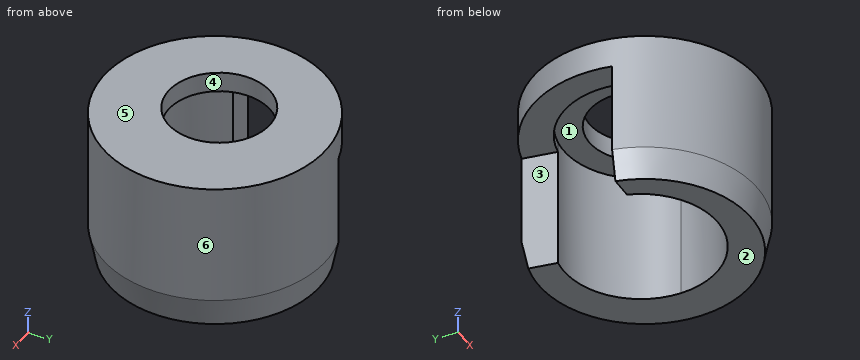
from build123d import *

# Parameters (mm, degrees)
F0_R     = 10.95
F1_DEPTH = 15
F3_DEPTH = 12
F4_DEPTH = 13
F6_D     = 10
F6_DEPTH = 10
F7_SIZE2 = 0.6
F7_SIZE  = 3


with BuildPart() as f1:
    # F0 (on Top) → F1 (new body)
    with BuildSketch(Plane.XY):
        Circle(F0_R)
    extrude(amount=F1_DEPTH)

    # F2 (on face) → F3 (cut)
    with BuildSketch(Plane(origin=(0, 0, 0), x_dir=(1, 0, 0), z_dir=(0, 0, -1))):
        with BuildLine():
            ThreePointArc((-2.024549, -7.399357), (-7.222314, -3.873485), (-7.916064, 2.368889))
            Line((-7.916064, 2.368889), (-10.690691, 2.368889))
            ThreePointArc((-10.690691, 2.368889), (-9.295049, -5.788313), (-2.590118, -10.639257))
            Line((-2.590118, -10.639257), (-2.024549, -7.399357))
        make_face()
    extrude(amount=-F3_DEPTH, mode=Mode.SUBTRACT)

    # F2 (on face) → F4 (cut)
    with BuildSketch(Plane(origin=(0, 0, 0), x_dir=(1, 0, 0), z_dir=(0, 0, -1))):
        with BuildLine():
            ThreePointArc((-2.024549, -7.399357), (4.051076, -5.719883), (6.7, 0))
            ThreePointArc((6.7, 0), (0.3999, 7.403394), (-7.916064, 2.368889))
            ThreePointArc((-7.916064, 2.368889), (-7.222314, -3.873485), (-2.024549, -7.399357))
        make_face()
    extrude(amount=-F4_DEPTH, mode=Mode.SUBTRACT)

    # F6
    with Locations(Plane(origin=(0, 0, 13), x_dir=(1, 0, 0), z_dir=(0, 0, -1))):
        with Locations((-0.8, 0)):
            Hole(F6_D / 2, depth=F6_DEPTH)

    # F7
    f7_edges = [f1.edges().sort_by_distance(p)[0] for p in [
        (6.765379, 8.610003, 0),
        (1.19152, -10.88498, 0),
    ]]
    chamfer(f7_edges, length=F7_SIZE, length2=F7_SIZE2)


solid = f1.part
Model file for the job. Use its own axes, mm. Face numbers are marked on the shaded views. A direction names the side the tool comes from. Round coordinates to 2 decimals unless told otherwise and drop trailing zeros. Order: outer loops, then holes, each group sorted by start corner. A loop starts at its lowest first (then second) coordinate and runs counter-clockwise, first axis right, second up. Notation, with made-up numbers: M -40,29 L 8,29 A25 cw 8,43 Z; hole C 27.25,-9.5 d6. An arc over 180 degrees is marked long. Write each question's results on one line, items separated by ' | '. Start each with the question number.
(1) Two-plate mould, pull along Y, no slides. Class the marked faces 4, 5 and 6: pulls with the +Y half, pulls with the -Y half, needs draft (parallel to the pull), parting line crosses it, or undercut.
(2) Drop flat-ended pins along their axis: pin 1 (1 mm diameter, centred on y = 7, z = 10.5, fed in from +X); pin 2 (2 mm diameter, centred on x = -8.5, z = 10.5, fed in from +Y); pin 3 (8 mm diameter, centred on y = -8, z = 8, fed in from -X); pin 4 (1.5 mm diameter, centred on x = 1.5, y = 0, fed in from +Z). Give the stop position or say it passes through.
(3) Which spindle directions (+Z, -Z, +X, -X, +Y, -Y) get a long thin tool onto all of the face, cutting with end or side? Do the marked faces 1, 2 and 3. Say none if no direction does.
(4) Saw through at B-B, the plane z = 9. Give the cut face in (x, y), then the cut area to 3 significant figures.
(5) Probe probe 1 along Y at (x, z) = (5.5, 5); probe 2 along Y at (x, z) = (5.75, 6.75); probe 3 along Z at (x, y) = (0.5, -6). List the from-to ranges inside material, lowest first. Write a range as from..to.
(6) Saw through at A-A, the plane x = 0. Give the cut face in (y, z), then the cut area to 3 significant figures.
Established:
1) face 4: undercut | face 5: needs draft | face 6: parting line crosses it
2) pin 1: stops at x = 8.81 | pin 2: stops at y = -2.37 | pin 3: stops at x = -10.19 | pin 4: passes through
3) face 1: -Z | face 2: -Z, +X, -X, +Y, -Y | face 3: -Z, -X
4) outline: M -10.69,-2.37 A10.95 ccw long -2.59,10.64 L -2.02,7.4 A7.5 cw long -7.92,-2.37 Z | area: 157 mm^2
5) probe 1: y = -9.47..-4.07, 4.07..9.47 | probe 2: y = -9.32..-3.65, 3.65..9.32 | probe 3: z = 13..15
6) outline: M -10.95,3 L -10.35,0 L -7.46,0 L -7.46,13 L -4.94,13 L -4.94,15 L -10.95,15 Z; M 4.94,13 L 7.46,13 L 7.46,0 L 10.35,0 L 10.95,3 L 10.95,15 L 4.94,15 Z | area: 113 mm^2
